```python
from build123d import *

# Parameters (mm, degrees)
SKETCH1_W           = 81
SKETCH1_H           = 32
BOSS_EXTRUDE1_DEPTH = 10
SKETCH2_W           = 77.5
SKETCH2_H           = 28.5
CUT_EXTRUDE1_DEPTH  = 10
SKETCH3_W           = 7.5
SKETCH3_H           = 32
BOSS_EXTRUDE2_DEPTH = 1.5
SKETCH4_W           = 64
SKETCH4_H           = 1
CUT_EXTRUDE2_DEPTH  = 10
BOSS_EXTRUDE3_DEPTH = 10
BOSS_EXTRUDE4_DEPTH = 10
FILLET1_R           = 2
FILLET2_R           = 2
FILLET3_R           = 2
FILLET4_R           = 2
CUT_EXTRUDE3_DEPTH  = 0.75
SKETCH8_W           = 21.5
SKETCH8_H           = 5.5
CUT_EXTRUDE4_DEPTH  = 0.75
FILLET5_R           = 3.5
FILLET6_R           = 3.5


with BuildPart() as part:
    # Sketch1 → Boss-Extrude1 (new body)
    with BuildSketch(Plane(origin=(0, 0, 0), x_dir=(1, 0, 0), z_dir=(0, 1, 0))):
        with Locations((-86.056207425, -60.23876691)):
            Rectangle(SKETCH1_W, SKETCH1_H)
    extrude(amount=BOSS_EXTRUDE1_DEPTH)

    # Sketch2 → Cut-Extrude1 (cut)
    with BuildSketch(Plane(origin=(0, 10, 0), x_dir=(1, 0, 0), z_dir=(0, 1, 0))):
        with Locations((-86.056207425, -60.23876691)):
            Rectangle(SKETCH2_W, SKETCH2_H)
    extrude(amount=-CUT_EXTRUDE1_DEPTH, mode=Mode.SUBTRACT)

    # Sketch3 → Boss-Extrude2 (add)
    with BuildSketch(Plane(origin=(0, 0, 0), x_dir=(-1, 0, 0), z_dir=(0, -1, 0))):
        with Locations((61.056207425, -60.23876691)):
            Rectangle(SKETCH3_W, SKETCH3_H)
        with Locations((111.056207425, -60.23876691)):
            Rectangle(SKETCH3_W, SKETCH3_H)
    extrude(amount=-BOSS_EXTRUDE2_DEPTH)

    # Sketch4 → Cut-Extrude2 (cut)
    with BuildSketch(Plane(origin=(0, 10, 0), x_dir=(1, 0, 0), z_dir=(0, 1, 0))):
        with Locations((-86.056207425, -75.73876691)):
            Rectangle(SKETCH4_W, SKETCH4_H)
    extrude(amount=-CUT_EXTRUDE2_DEPTH, mode=Mode.SUBTRACT)

    # Sketch5 → Boss-Extrude3 (add)
    with BuildSketch(Plane(origin=(0, 10, 0), x_dir=(1, 0, 0), z_dir=(0, 1, 0))):
        Polygon((-116.976207425, -75.23876691), (-117.306207425, -76.781751031), (-115.806207425, -76.781751031), (-116.146207425, -75.23876691), align=None)
    extrude(amount=-BOSS_EXTRUDE3_DEPTH)

    # Sketch6 → Boss-Extrude4 (add)
    with BuildSketch(Plane(origin=(0, 10, 0), x_dir=(1, 0, 0), z_dir=(0, 1, 0))):
        Polygon((-55.966207425, -75.23876691), (-56.306207425, -76.781751031), (-54.806207425, -76.781751031), (-55.136207425, -75.23876691), align=None)
    extrude(amount=-BOSS_EXTRUDE4_DEPTH)

    # Fillet1
    fillet1_edges = [part.edges().sort_by_distance(p)[0] for p in [
        (-126.556207425, 5, 76.23876691),
    ]]
    fillet(fillet1_edges, radius=FILLET1_R)

    # Fillet2
    fillet2_edges = [part.edges().sort_by_distance(p)[0] for p in [
        (-45.556207425, 5, 76.23876691),
    ]]
    fillet(fillet2_edges, radius=FILLET2_R)

    # Fillet3
    fillet3_edges = [part.edges().sort_by_distance(p)[0] for p in [
        (-45.556207425, 5, 44.23876691),
    ]]
    fillet(fillet3_edges, radius=FILLET3_R)

    # Fillet4
    fillet4_edges = [part.edges().sort_by_distance(p)[0] for p in [
        (-126.556207425, 5, 44.23876691),
    ]]
    fillet(fillet4_edges, radius=FILLET4_R)

    # Sketch7 → Cut-Extrude3 (cut)
    with BuildSketch(Plane.XY.offset(75.23876691)):
        with BuildLine():
            Line((-111.806207425, 10), (-106.806207425, 10))
            Line((-106.806207425, 10), (-106.806207425, 3.5))
            ThreePointArc((-106.806207425, 3.5), (-107.391993862, 2.085786438), (-108.806207425, 1.5))
            Line((-108.806207425, 1.5), (-109.806207425, 1.5))
            ThreePointArc((-109.806207425, 1.5), (-111.220420987, 2.085786438), (-111.806207425, 3.5))
            Line((-111.806207425, 3.5), (-111.806207425, 10))
        make_face()
        with BuildLine():
            Line((-65.306207425, 10), (-60.306207425, 10))
            Line((-60.306207425, 10), (-60.306207425, 3.5))
            ThreePointArc((-60.306207425, 3.5), (-60.891993862, 2.085786438), (-62.306207425, 1.5))
            Line((-62.306207425, 1.5), (-63.306207425, 1.5))
            ThreePointArc((-63.306207425, 1.5), (-64.720420987, 2.085786438), (-65.306207425, 3.5))
            Line((-65.306207425, 3.5), (-65.306207425, 10))
        make_face()
        with BuildLine():
            Line((-104.306207425, 10), (-99.306207425, 10))
            Line((-99.306207425, 10), (-99.306207425, 3.5))
            ThreePointArc((-99.306207425, 3.5), (-99.891993862, 2.085786438), (-101.306207425, 1.5))
            Line((-101.306207425, 1.5), (-102.306207425, 1.5))
            ThreePointArc((-102.306207425, 1.5), (-103.720420987, 2.085786438), (-104.306207425, 3.5))
            Line((-104.306207425, 3.5), (-104.306207425, 10))
        make_face()
        with BuildLine():
            Line((-72.806207425, 10), (-67.806207425, 10))
            Line((-67.806207425, 10), (-67.806207425, 3.5))
            ThreePointArc((-67.806207425, 3.5), (-68.391993862, 2.085786438), (-69.806207425, 1.5))
            Line((-69.806207425, 1.5), (-70.806207425, 1.5))
            ThreePointArc((-70.806207425, 1.5), (-72.220420987, 2.085786438), (-72.806207425, 3.5))
            Line((-72.806207425, 3.5), (-72.806207425, 10))
        make_face()
    extrude(amount=-CUT_EXTRUDE3_DEPTH, mode=Mode.SUBTRACT)

    # Sketch8 → Cut-Extrude4 (cut)
    with BuildSketch(Plane.XY.offset(75.23876691)):
        with Locations((-86.056207425, 2.75)):
            Rectangle(SKETCH8_W, SKETCH8_H)
    extrude(amount=-CUT_EXTRUDE4_DEPTH, mode=Mode.SUBTRACT)

    # Fillet5
    fillet5_edges = [part.edges().sort_by_distance(p)[0] for p in [
        (-96.806207425, 5.5, 74.86376691),
    ]]
    fillet(fillet5_edges, radius=FILLET5_R)

    # Fillet6
    fillet6_edges = [part.edges().sort_by_distance(p)[0] for p in [
        (-75.306207425, 5.5, 74.86376691),
    ]]
    fillet(fillet6_edges, radius=FILLET6_R)


solid = part.part
```
Part model, mm, in its own coordinate system. A direction names the side the tool comes from. Round coordinates to 2 decimals unless told otherwise and drop trailing zeros. Loops run counter-clockwise (first coordinate to the right, second up) from the corner with the lowest first, then second, coordinate; pieces in that order, holes last. Notation, with made-up numbers: (-5.5, 9) -> (20.5, 9) arc R10 cw to (20.5, 27) -> close; hole circle Ø7 at (25, -9.75). An arc over 180 degrees is marked (long way). Use a Markdown table: item, result.
1) Cut at C-C, the plane y = 4.25. State how many separate pieces and enclosed holes the cut face has, and give its area (3 significant figures).
The answers:
| item | result |
|---|---|
| separate pieces | 5 |
| enclosed holes | 0 |
| area | 290 mm2 |
2) Pull direction X, two halves, no side cores. Call faces 1 (the flat face through (-117, 5, 76.782)), 2 (the cylindrical face through (-125.955, 5.07, 44.809)), 3 (the flat face through (-86, 6, 74.489)): pulls with the +X half, pulls with the -X half, needs draft (parallel to the pull), parting line crosses it, or undercut.
The answers:
| item | result |
|---|---|
| face 1 | needs draft |
| face 2 | pulls with the -X half |
| face 3 | undercut |
3) Drop flat-ended pins along their axis: pin 1 Ø12 at (x, z) = (-94.5, 73) entering from -Y; pin 2 Ø0.8 at (x, z) = (-89.5, 74.5) entering from -Y; pin 3 Ø4 at (x, y) = (-107.5, 8.5) entering from +Z; pin 4 Ø0.6 at (y, z) = (0.5, 75) entering from -X. Give the stop position or say it passes through.
The answers:
| item | result |
|---|---|
| pin 1 | stops at y = 0 |
| pin 2 | stops at y = 5.5 |
| pin 3 | stops at z = 75.24 |
| pin 4 | stops at x = -126.5 |
4) Cut at D-D, the plane x = -61.5. List the corners of the cut face in (y, z).
The answers:
| item | result |
|---|---|
| outline | (0, 44.24) -> (10, 44.24) -> (10, 45.99) -> (1.5, 45.99) -> (1.5, 74.49) -> (1.67, 74.49) -> (1.67, 75.24) -> (0, 75.24) -> close |
5) Cut at B-B, the plane z = 49. List the corners of the cut face in (x, y), and give its area (3 significant figures).
The answers:
| item | result |
|---|---|
| outline | (-126.56, 0) -> (-124.81, 0) -> (-124.81, 10) -> (-126.56, 10) -> close; (-114.81, 0) -> (-107.31, 0) -> (-107.31, 1.5) -> (-114.81, 1.5) -> close; (-64.81, 0) -> (-57.31, 0) -> (-57.31, 1.5) -> (-64.81, 1.5) -> close; (-47.31, 0) -> (-45.56, 0) -> (-45.56, 10) -> (-47.31, 10) -> close |
| area | 57.5 mm2 |
6) Tool access for faces 4 (the flat face through (-51, 5, 76.239)), 5 (the flat face through (-114.806, 1, 60)), 6 (the flat face through (-121, 5, 76.239)), 7 (the cylindrical face through (-60.88, 2.1, 74.87)): list every direction of +Z, -Z, +X, -X, +Y, -Y with a clear straight run to the whole face (end or side of a thin tool).
The answers:
| item | result |
|---|---|
| face 4 | +Z, +X, +Y, -Y |
| face 5 | +Y, -Y |
| face 6 | +Z, -X, +Y, -Y |
| face 7 | +Z, +Y |
7) Probe line 1 (X direction, y = 1, z = 52); line 2 (Z direction, x = -121.5, y = 6); line 3 (X direction, y = 8.75, z = 72). List the from-to ranges inside material, lowest first. Write a range as [from, to].
The answers:
| item | result |
|---|---|
| line 1 | x = [-126.56, -124.81], [-114.81, -107.31], [-64.81, -57.31], [-47.31, -45.56] |
| line 2 | z = [44.24, 45.99], [74.49, 76.24] |
| line 3 | x = [-126.56, -124.81], [-47.31, -45.56] |
8) Cut at A-A, the plane x = -92. List the corners of the cut face in (y, z), and give its area (3 significant figures).
The answers:
| item | result |
|---|---|
| outline | (0, 44.24) -> (10, 44.24) -> (10, 45.99) -> (0, 45.99) -> close; (5.5, 74.49) -> (10, 74.49) -> (10, 75.24) -> (5.5, 75.24) -> close |
| area | 20.9 mm2 |
